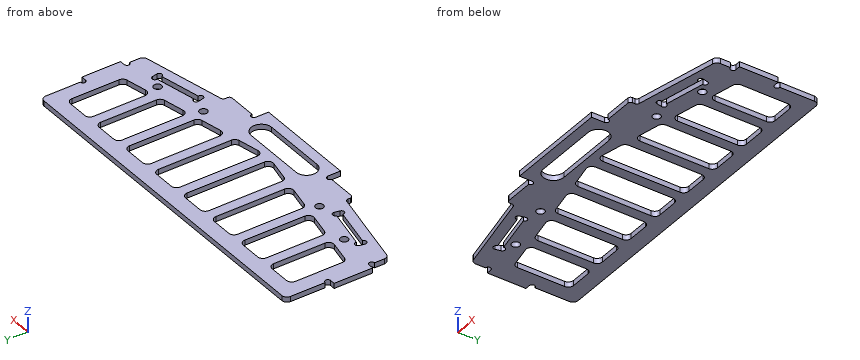
```python
from build123d import *

# Parameters (mm, degrees)
SKETCH_1_W           = 136
SKETCH_1_H           = 50
EXTRUDE_1_DEPTH      = 2
SKETCH_2_W           = 4
SKETCH_2_H           = 15
EXTRUDE_2_DEPTH      = 2
SKETCH_3_R           = 1.05
CUT_EXTRUDE_1_DEPTH  = 2
CUT_EXTRUDE_3_DEPTH  = 2
SKETCH_5_R           = 1.05
CUT_EXTRUDE_4_DEPTH  = 10
SKETCH_6_R           = 1.05
CUT_EXTRUDE_5_DEPTH  = 10
SKETCH_7_W           = 40
SKETCH_7_H           = 10
EXTRUDE_3_DEPTH      = 2
SKETCH_8_R           = 1.05
CUT_EXTRUDE_6_DEPTH  = 10
SKETCH_9_R           = 1.525
CUT_EXTRUDE_7_DEPTH  = 22
CUT_EXTRUDE_8_DEPTH  = 22
FILLET_1_R           = 1.1
FILLET_2_R           = 2
CUT_EXTRUDE_9_DEPTH  = 22
FILLET_3_R           = 2
CUT_EXTRUDE_10_DEPTH = 2


with BuildPart() as part:
    # 草图1 → 凸台-拉伸1 (new body)
    with BuildSketch(Plane.XY):
        Rectangle(SKETCH_1_W, SKETCH_1_H)
    extrude(amount=EXTRUDE_1_DEPTH)

    # 草图2 → 凸台-拉伸2 (add)
    with BuildSketch(Plane.XY.offset(2)):
        with Locations((68, 0)):
            Rectangle(SKETCH_2_W, SKETCH_2_H)
    extrude_2 = extrude(amount=-EXTRUDE_2_DEPTH)

    # 镜向1: 凸台-拉伸2 across plane
    add(extrude_2.mirror(Plane(origin=(0, 0, 0), x_dir=(0, 0, 1), z_dir=(1, 0, 0))))

    # 草图3 → 切除-拉伸1 (cut)
    with BuildSketch(Plane(origin=(0, 0, 0), x_dir=(-1, 0, 0), z_dir=(0, 0, -1))):
        with Locations((68, 8.55)):
            Circle(SKETCH_3_R)
        with Locations((68, -8.55)):
            Circle(SKETCH_3_R)
        with Locations((-68, 8.55)):
            Circle(SKETCH_3_R)
        with Locations((-68, -8.55)):
            Circle(SKETCH_3_R)
    extrude(amount=-CUT_EXTRUDE_1_DEPTH, mode=Mode.SUBTRACT)

    # 草图4 → 切除-拉伸3 (cut)
    with BuildSketch(Plane.XY.offset(2)):
        Polygon((38.094522867, -17.190550425), (57.770246389, -13.082521228), (57.341049309, -11.026848621), (37.665325786, -15.134877819), align=None)
    cut_extrude_3 = extrude(amount=-CUT_EXTRUDE_3_DEPTH, mode=Mode.SUBTRACT)

    # 草图5 → 切除-拉伸4 (cut)
    with BuildSketch(Plane.XY.offset(2)):
        with Locations((39.12235917, -16.975951885)):
            Circle(SKETCH_5_R)
        with Locations((56.742410085, -13.297119768)):
            Circle(SKETCH_5_R)
    cut_extrude_4 = extrude(amount=-CUT_EXTRUDE_4_DEPTH, mode=Mode.SUBTRACT)

    # 草图6 → 切除-拉伸5 (cut)
    with BuildSketch(Plane.XY.offset(2)):
        with Locations((38.69316209, -14.920279278)):
            Circle(SKETCH_6_R)
        with Locations((56.313213005, -11.241447162)):
            Circle(SKETCH_6_R)
    cut_extrude_5 = extrude(amount=-CUT_EXTRUDE_5_DEPTH, mode=Mode.SUBTRACT)

    # 镜向2: 切除-拉伸3, 切除-拉伸4, 切除-拉伸5 across plane
    add(cut_extrude_3.mirror(Plane(origin=(0, 0, 0), x_dir=(0, 0, 1), z_dir=(1, 0, 0))), mode=Mode.SUBTRACT)
    add(cut_extrude_4.mirror(Plane(origin=(0, 0, 0), x_dir=(0, 0, 1), z_dir=(1, 0, 0))), mode=Mode.SUBTRACT)
    add(cut_extrude_5.mirror(Plane(origin=(0, 0, 0), x_dir=(0, 0, 1), z_dir=(1, 0, 0))), mode=Mode.SUBTRACT)

    # 草图7 → 凸台-拉伸3 (add)
    with BuildSketch(Plane.XY.offset(2)):
        with Locations((0, -25)):
            Rectangle(SKETCH_7_W, SKETCH_7_H)
    extrude(amount=-EXTRUDE_3_DEPTH)

    # 草图8 → 切除-拉伸6 (cut)
    with BuildSketch(Plane(origin=(0, 0, 0), x_dir=(-1, 0, 0), z_dir=(0, 0, -1))):
        with Locations((21.05, -25)):
            Circle(SKETCH_8_R)
        with Locations((-21.05, -25)):
            Circle(SKETCH_8_R)
    extrude(amount=-CUT_EXTRUDE_6_DEPTH, mode=Mode.SUBTRACT)

    # 草图9 → 切除-拉伸7 (cut)
    with BuildSketch(Plane(origin=(0, 0, 0), x_dir=(-1, 0, 0), z_dir=(0, 0, -1))):
        with Locations((-51.794726427, -9.171234843)):
            Circle(SKETCH_9_R)
        with Locations((-32.216892077, -13.258826084)):
            Circle(SKETCH_9_R)
    cut_extrude_7 = extrude(amount=-CUT_EXTRUDE_7_DEPTH, mode=Mode.SUBTRACT)

    # 镜向3: 切除-拉伸7 across plane
    add(cut_extrude_7.mirror(Plane(origin=(0, 0, 0), x_dir=(0, 0, 1), z_dir=(1, 0, 0))), mode=Mode.SUBTRACT)

    # 草图10 → 切除-拉伸8 (cut)
    with BuildSketch(Plane(origin=(0, 0, 0), x_dir=(-1, 0, 0), z_dir=(0, 0, -1))):
        Polygon((-68, -15.032938627), (-34.1, -22.110807434), (-34.1, -25), (-68, -25), align=None)
    cut_extrude_8 = extrude(amount=-CUT_EXTRUDE_8_DEPTH, mode=Mode.SUBTRACT)

    # 镜向4: 切除-拉伸8 across plane
    add(cut_extrude_8.mirror(Plane(origin=(0, 0, 0), x_dir=(0, 0, 1), z_dir=(1, 0, 0))), mode=Mode.SUBTRACT)

    # 圆角1
    fillet_1_edges = [part.edges().sort_by_distance(p)[0] for p in [
        (34.1, -25, 1),
        (34.1, -22.110807434, 1),
        (-34.1, -25, 1),
        (-34.1, -22.110807434, 1),
    ]]
    fillet(fillet_1_edges, radius=FILLET_1_R)

    # 圆角2
    fillet_2_edges = [part.edges().sort_by_distance(p)[0] for p in [
        (68, -15.032938627, 1),
        (-68, -15.032938627, 1),
        (-68, 25, 1),
        (68, 25, 1),
    ]]
    fillet(fillet_2_edges, radius=FILLET_2_R)

    # 草图11 → 切除-拉伸9 (cut)
    with BuildSketch(Plane(origin=(0, 0, 0), x_dir=(-1, 0, 0), z_dir=(0, 0, -1))):
        Polygon((14, 19), (2, 19), (2, -15.481457178), (14, -12.976016892), align=None)
        Polygon((30, 19), (18, 19), (18, -12.14087013), (30, -9.635429844), align=None)
        Polygon((46, 19), (34, 19), (34, -8.800283082), (46, -6.294842797), align=None)
        Polygon((62, 19), (50, 19), (50, -5.459696035), (62, -2.954255749), align=None)
    cut_extrude_9 = extrude(amount=-CUT_EXTRUDE_9_DEPTH, mode=Mode.SUBTRACT)

    # 镜向5: 切除-拉伸9 across plane
    add(cut_extrude_9.mirror(Plane(origin=(0, 0, 0), x_dir=(0, 0, 1), z_dir=(1, 0, 0))), mode=Mode.SUBTRACT)

    # 圆角3
    fillet_3_edges = [part.edges().sort_by_distance(p)[0] for p in [
        (-14, 19, 1),
        (-14, -12.976016892, 1),
        (-2, -15.481457178, 1),
        (-2, 19, 1),
        (-30, 19, 1),
        (-30, -9.635429844, 1),
        (-18, -12.14087013, 1),
        (-18, 19, 1),
        (-46, 19, 1),
        (-46, -6.294842797, 1),
        (-34, -8.800283082, 1),
        (-34, 19, 1),
        (-50, 19, 1),
        (-62, 19, 1),
        (-62, -2.954255749, 1),
        (-50, -5.459696035, 1),
        (14, -12.976016892, 1),
        (14, 19, 1),
        (2, 19, 1),
        (2, -15.481457178, 1),
        (30, -9.635429844, 1),
        (30, 19, 1),
        (18, 19, 1),
        (18, -12.14087013, 1),
        (46, -6.294842797, 1),
        (46, 19, 1),
        (34, 19, 1),
        (34, -8.800283082, 1),
        (62, 19, 1),
        (50, 19, 1),
        (50, -5.459696035, 1),
        (62, -2.954255749, 1),
    ]]
    fillet(fillet_3_edges, radius=FILLET_3_R)

    # 草图12 → 切除-拉伸10 (cut)
    with BuildSketch(Plane(origin=(0, 0, 0), x_dir=(-1, 0, 0), z_dir=(0, 0, -1))):
        with BuildLine():
            Line((-12.5, -18.020756897), (12.5, -18.020756897))
            ThreePointArc((12.5, -18.020756897), (16.489621551, -22.010378449), (12.5, -26))
            Line((12.5, -26), (-12.5, -26))
            ThreePointArc((-12.5, -26), (-16.489621551, -22.010378449), (-12.5, -18.020756897))
        make_face()
    extrude(amount=-CUT_EXTRUDE_10_DEPTH, mode=Mode.SUBTRACT)


solid = part.part
```
CAD build for the part. Positions are in the model's coordinates, mm. Give positions to 0.01 mm unless a question says otherwise; leave off trailing zeros. Order: outer loops, then holes, each group sorted by start corner. A loop starts at its lowest first (then second) coordinate and runs counter-clockwise, first axis right, second up. Notation, with made-up numbers: M 28.5,-20.5 L 71.5,-20.5 A24 cw 71.5,7.5 Z; hole C 10.5,53 d3. An arc over 180 degrees is marked long. Put each result on its own line as item: value. Start each with the question number.
(1) Saw through at B-B, the plane y = 15.5. Give the number of separate pieces and of enclosed holes in the cut face, then the cut area to 3 significant figures.
(2) Flat gauge pins, fed straight in: pin 1 Ø1 at (x, z) = (31.5, 1.5) entering from -Y; pin 2 Ø0.7 at (y, z) = (-23.5, 1) entering from +X; pin 3 Ø0.6 at (y, z) = (8, 0.5) entering from +X. Where does each tip first touch, or does it go through?
(3) Saw through at A-A, the plane x = 24. Write the cut outline in (y, z), then the cut area to 3 significant figures.
(4) Saw through at C-C, the plane y = -20. Write the cut outline in (x, z), then the cut area to 3 significant figures.
(5) Drill centre lines: line 1 along Y through (x, z) = (12, 0.75); line 2 along Y through (x, z) = (-53, 0.8); line 3 along Y through (x, z) = (-40.5, 0.45). Where is each one in solid material? Low to high.
Check result:
1. separate pieces: 9
1. enclosed holes: 0
1. area: 80.0 mm2
2. pin 1: stops at y = -25
2. pin 2: stops at x = 34.1
2. pin 3: stops at x = 67.38
3. outline: M -25,0 L -10.89,0 L -10.89,2 L -25,2 Z; M 19,0 L 25,0 L 25,2 L 19,2 Z
3. area: 40.2 mm2
4. outline: M -44.21,0 L -15.95,0 L -15.95,2 L -44.21,2 Z; M 15.95,0 L 44.21,0 L 44.21,2 L 15.95,2 Z
4. area: 113 mm2
5. line 1: y = -30 to -26, -18.02 to -13.39, 19 to 25
5. line 2: y = -18.16 to -14.08, -11.93 to -10.11, -8.24 to -4.83, 19 to 25
5. line 3: y = -20.77 to -16.69, -14.54 to -7.44, 19 to 25
